Source: CAD feature listing. Evaluate the final solid. Frame: model axes, mm. A direction names the side the tool comes from. Coordinates: 2 decimals unless noted, no trailing zeros. Order: outer loops, then holes, each group sorted by start corner. A loop starts at its lowest first (then second) coordinate and runs counter-clockwise, first axis right, second up.
```python
from build123d import *

# Parameters (mm, degrees)
CROQUIS1_W              = 20
CROQUIS1_H              = 25
SALIENTE_EXTRUIR4_DEPTH = 16
CORTAR_EXTRUIR1_START   = 10
CROQUIS4_W              = 21
CROQUIS4_H              = 12
CORTAR_EXTRUIR1_DEPTH   = 18
SALIENTE_EXTRUIR6_START = -10
CROQUIS5_W              = 21
CROQUIS5_H              = 1
SALIENTE_EXTRUIR6_DEPTH = 16
SALIENTE_EXTRUIR7_START = 10
CROQUIS7_W              = 2
CROQUIS7_H              = 8
SALIENTE_EXTRUIR7_DEPTH = 4
CORTAR_EXTRUIR2_START   = 14
CROQUIS7_2_W            = 2
CROQUIS7_2_H            = 8
CORTAR_EXTRUIR2_DEPTH   = 8
CROQUIS8_W              = 12.75
CROQUIS8_H              = 11
SALIENTE_EXTRUIR8_DEPTH = 3
CROQUIS9_W              = 9.75
CROQUIS9_H              = 1.5
CORTAR_EXTRUIR4_DEPTH   = 21.5


with BuildPart() as part:
    # Croquis1 → Saliente-Extruir4 (new body)
    with BuildSketch(Plane(origin=(0, 0, 0), x_dir=(1, 0, 0), z_dir=(0, 1, 0))):
        Rectangle(CROQUIS1_W, CROQUIS1_H)
    extrude(amount=SALIENTE_EXTRUIR4_DEPTH)

    # Croquis4 → Cortar-Extruir1 (cut)
    with BuildSketch(Plane(origin=(0, 0, 0), x_dir=(0, 0, -1), z_dir=(1, 0, 0)).offset(CORTAR_EXTRUIR1_START)):
        with Locations((0, 8)):
            Rectangle(CROQUIS4_W, CROQUIS4_H)
    extrude(amount=-CORTAR_EXTRUIR1_DEPTH, mode=Mode.SUBTRACT)

    # Croquis5 → Saliente-Extruir6 (add)
    with BuildSketch(Plane(origin=(0, 0, 0), x_dir=(0, 0, -1), z_dir=(1, 0, 0)).offset(SALIENTE_EXTRUIR6_START)):
        with Locations((0, 8)):
            Rectangle(CROQUIS5_W, CROQUIS5_H)
    extrude(amount=SALIENTE_EXTRUIR6_DEPTH)

    # Croquis7 → Saliente-Extruir7 (add)
    with BuildSketch(Plane(origin=(0, 0, 0), x_dir=(0, 0, -1), z_dir=(1, 0, 0)).offset(SALIENTE_EXTRUIR7_START)):
        with Locations((-11.5, 8)):
            Rectangle(CROQUIS7_W, CROQUIS7_H)
        with Locations((11.5, 8)):
            Rectangle(CROQUIS7_W, CROQUIS7_H)
    extrude(amount=SALIENTE_EXTRUIR7_DEPTH)

    # Croquis7<2> → Cortar-Extruir2 (cut)
    with BuildSketch(Plane(origin=(0, 0, 0), x_dir=(0, 0, -1), z_dir=(1, 0, 0)).offset(CORTAR_EXTRUIR2_START)):
        with Locations((-11.5, 8)):
            Rectangle(CROQUIS7_2_W, CROQUIS7_2_H)
        with Locations((11.5, 8)):
            Rectangle(CROQUIS7_2_W, CROQUIS7_2_H)
    extrude(amount=-CORTAR_EXTRUIR2_DEPTH, mode=Mode.SUBTRACT)

    # Croquis8 → Saliente-Extruir8 (add)
    with BuildSketch(Plane(origin=(0, 0, 0), x_dir=(1, 0, 0), z_dir=(0, 1, 0))):
        with Locations((-3.625, 0)):
            Rectangle(CROQUIS8_W, CROQUIS8_H)
    extrude(amount=-SALIENTE_EXTRUIR8_DEPTH)

    # Croquis9 → Cortar-Extruir4 (cut, symmetric)
    with BuildSketch(Plane.XY):
        with Locations((-3.625, -0.75)):
            Rectangle(CROQUIS9_W, CROQUIS9_H)
    extrude(amount=CORTAR_EXTRUIR4_DEPTH, both=True, mode=Mode.SUBTRACT)


solid = part.part
```
Q1. Section query B-B on z = -0.5. Output: boundary loops of the cut face in (x, y), plus the area to 3 significant figures.
Solutions:
outline: (-10, -3) - (2.75, -3) - (2.75, 0) - (10, 0) - (10, 2) - (-8, 2) - (-8, 7.5) - (6, 7.5) - (6, 8.5) - (-8, 8.5) - (-8, 14) - (10, 14) - (10, 16) - (-10, 16) - close; hole (-8.5, -1.5) - (1.25, -1.5) - (1.25, 0) - (-8.5, 0) - close
area: 142 mm2
Q2. Pull-direction query (Z, two-part tool) for faces 5 (the flat face through (0, 8, -12.5)), 6 (the flat face through (-4, -1.5, 0)), 7 (the flat face through (-1, 7.5, 0)); classes: pulls with the +Z half, pulls with the -Z half, needs draft (parallel to the pull), parting line crosses it, or undercut.
Solutions:
face 5: pulls with the -Z half
face 6: needs draft
face 7: undercut
Q3. Set-up query: faces 1 (the flat face through (8, 12, -11)), 2 (the flat face through (-8.5, -1, 0)), 3 (the flat face through (1, 2, 0)), 4 (the flat face through (-4, -3, 0)). Return all of +Z, -Z, +X, -X, +Y, -Y with unobstructed straight access to the full face (end or side cutting, diameter ignored); none if empty.
Solutions:
face 1: +Z, -Z, +X
face 2: +Z, -Z
face 3: +X
face 4: +Z, -Z, +X, -X, -Y
Q4. Section query C-C on x = 8.75. Output: boundary loops of the cut face in (y, z), plus the area to 3 significant figures.
Solutions:
outline: (0, -12.5) - (4, -12.5) - (4, -10.5) - (2, -10.5) - (2, 10.5) - (4, 10.5) - (4, 12.5) - (0, 12.5) - close; (12, -12.5) - (16, -12.5) - (16, 12.5) - (12, 12.5) - (12, 10.5) - (14, 10.5) - (14, -10.5) - (12, -10.5) - close
area: 116 mm2
Q5. Section query A-A on x = -1. Output: boundary loops of the cut face in (y, z).
Solutions:
outline: (-3, -5.5) - (-1.5, -5.5) - (-1.5, 5.5) - (-3, 5.5) - close; (0, -12.5) - (16, -12.5) - (16, 12.5) - (0, 12.5) - close; hole (2, -10.5) - (7.5, -10.5) - (7.5, 10.5) - (2, 10.5) - close; hole (8.5, -10.5) - (14, -10.5) - (14, 10.5) - (8.5, 10.5) - close
Q6. Pin query (flat end, axial travel): P1, Ø6.5, axis at y = 6.5, z = -4, coming from the +X side; P2, Ø1.5, axis at y = 9.5, z = 3.5, coming from the +X side; P3, Ø1.5, axis at y = -1.5, z = 2.5, coming from the +X side. Return the tip coordinate at first contact, or that it passes through.
Solutions:
P1: stops at x = 6
P2: stops at x = -8
P3: stops at x = 2.75
Q7. Section query D-D on y = 6.75. Output: boundary loops of the cut face in (x, z).
Solutions:
outline: (-10, -12.5) - (6, -12.5) - (6, -10.5) - (-8, -10.5) - (-8, 10.5) - (6, 10.5) - (6, 12.5) - (-10, 12.5) - close
Q8. Material intervals for line 1 along Y through (x, z) = (5, -3.75); line 2 along Y through (x, z) = (-7.75, 3.5); line 3 along Z through (x, y) = (7.25, 12.25), sorted ascending.
Solutions:
line 1: y = 0 to 2, 7.5 to 8.5, 14 to 16
line 2: y = -3 to -1.5, 0 to 2, 7.5 to 8.5, 14 to 16
line 3: z = -12.5 to -10.5, 10.5 to 12.5
